Can you work these out from the drawing? Everything is in mm from the part's minimum corner. A direction names the side the tool comes from. Round coordinates to 2 decimals unless told otherwise and drop trailing zeros. Loops run counter-clockwise (first coordinate to the right, second up) from the corner with the lowest first, then second, coordinate; pieces in that order, holes last. Notation, with made-up numbers: M 33.25,-21.5 L 60.25,-21.5 A19 cw 60.25,-12.5 Z; hole C 29.25,73 d4. An arc over 180 degrees is marked long. Answer in a Markdown table with one row per item.
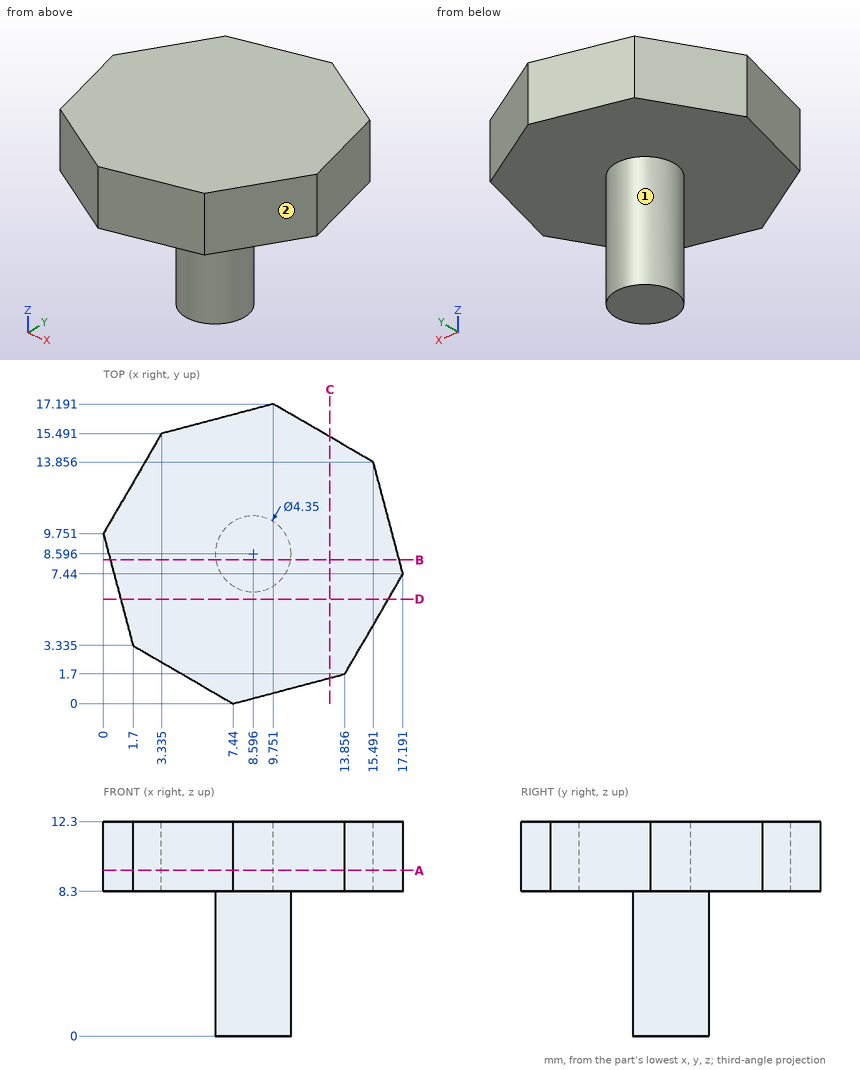
1) I want a section at B-B, the plane y = 8.25. Please give me the cut outline in (x, z).
Computed:
| item | result |
|---|---|
| outline | M 0.4,8.3 L 6.45,8.3 L 6.45,0 L 10.74,0 L 10.74,8.3 L 16.98,8.3 L 16.98,12.3 L 0.4,12.3 Z |
2) Which directions (+Z, -Z, +X, -X, +Y, -Y) give clear straight access to the entire face, cutting with the end or side of a thin tool? Please do the marked faces 1 and 2.
Computed:
| item | result |
|---|---|
| face 1 | -Z |
| face 2 | +Z, -Z, +X, -Y |
3) Will these pins go through, and if not, where does the flat tip stop? P1, Ø2, axis at y = 11, z = 7, coming from the +X side (1 decimal); P2, Ø6, axis at y = 12, z = 10, coming from the +X side; P3, Ø3, axis at x = 4.5, z = 11, coming from the +Y side.
Computed:
| item | result |
|---|---|
| P1 | stops at x = 10.3 |
| P2 | stops at x = 16.78 |
| P3 | stops at y = 16.2 |
4) I want a section at A-A, the plane z = 9.5. Please give me the cut outline in (x, y) (1 decimal).
Computed:
| item | result |
|---|---|
| outline | M 0,9.8 L 1.7,3.3 L 7.4,0 L 13.9,1.7 L 17.2,7.4 L 15.5,13.9 L 9.8,17.2 L 3.3,15.5 Z |
5) I want a section at C-C, the plane x = 13. Please give me the cut outline in (y, z).
Computed:
| item | result |
|---|---|
| outline | M 1.47,8.3 L 15.3,8.3 L 15.3,12.3 L 1.47,12.3 Z |
6) I want a section at D-D, the plane y = 6. Please give me the cut outline in (x, z) (1 decimal).
Computed:
| item | result |
|---|---|
| outline | M 1,8.3 L 16.4,8.3 L 16.4,12.3 L 1,12.3 Z |
7) I need wall thicknesses on line 1 (Y direction, x = 8.75, z = 2) (1 decimal); line 2 (Z direction, x = 13, y = 3.5); line 3 (Y direction, x = 4.75, z = 11.75) (1 decimal). Which ranges of each line are inside material? Lowest first, please.
Computed:
| item | result |
|---|---|
| line 1 | y = 6.4 to 10.8 |
| line 2 | z = 8.3 to 12.3 |
| line 3 | y = 1.6 to 15.9 |
